```python
from build123d import *

# Parameters (mm, degrees)
SKETCH1_W           = 65
SKETCH1_H           = 30
BOSS_EXTRUDE1_DEPTH = 58
FILLET1_R           = 13
SKETCH15_W          = 83.696095513
SKETCH15_H          = 31.69844841
CUT_EXTRUDE7_DEPTH  = 50
SKETCH18_R          = 16
CUT_EXTRUDE10_DEPTH = 5.5
CUT_EXTRUDE12_REACH = 90.397
SKETCH3_R           = 1.6
SKETCH21_W          = 2
SKETCH21_H          = 2
CUT_EXTRUDE13_DEPTH = 8


with BuildPart() as part:
    # Sketch1 → Boss-Extrude1 (new body)
    with BuildSketch(Plane(origin=(0, 0, 0), x_dir=(1, 0, 0), z_dir=(0, 1, 0))):
        with Locations((7.5, 0)):
            Rectangle(SKETCH1_W, SKETCH1_H)
    extrude(amount=BOSS_EXTRUDE1_DEPTH)

    # Fillet1
    fillet1_edges = [part.edges().sort_by_distance(p)[0] for p in [
        (40, 29, 15),
        (-25, 29, 15),
        (-25, 29, -15),
        (40, 29, -15),
    ]]
    fillet(fillet1_edges, radius=FILLET1_R)

    # Sketch15 → Cut-Extrude7 (cut)
    with BuildSketch(Plane(origin=(0, -10, 0), x_dir=(-1, 0, 0), z_dir=(0, -1, 0))):
        with Locations((-0.057440767, 0.030479277)):
            Rectangle(SKETCH15_W, SKETCH15_H)
    extrude(amount=-CUT_EXTRUDE7_DEPTH, mode=Mode.SUBTRACT)

    # Sketch18 → Cut-Extrude10 (cut)
    with BuildSketch(Plane(origin=(0, 58, 0), x_dir=(1, 0, 0), z_dir=(0, 1, 0))):
        with Locations((6.828508286, 0)):
            Circle(SKETCH18_R)
    extrude(amount=-CUT_EXTRUDE10_DEPTH, mode=Mode.SUBTRACT)

    # Sketch3 → Cut-Extrude12 (cut, up to next)
    with BuildSketch(Plane.ZY.offset(25), mode=Mode.PRIVATE) as cut_extrude12_sk1:
        with Locations((0, 50.4)):
            Circle(SKETCH3_R)
    cut_extrude12_tool1 = extrude(cut_extrude12_sk1.sketch, amount=-CUT_EXTRUDE12_REACH, mode=Mode.PRIVATE) & part.part
    add(cut_extrude12_tool1.solids().sort_by_distance((-25, 50.4, 0))[0], mode=Mode.SUBTRACT)

    # Sketch21 → Cut-Extrude13 (cut)
    with BuildSketch(Plane(origin=(0, 52.5, 0), x_dir=(1, 0, 0), z_dir=(0, 1, 0))):
        with Locations((6.828508286, 0)):
            Rectangle(SKETCH21_W, SKETCH21_H)
    extrude(amount=-CUT_EXTRUDE13_DEPTH, mode=Mode.SUBTRACT)

    # Sketch24 → Revolve1 (revolve)
    with BuildSketch(Plane.XY, mode=Mode.PRIVATE) as revolve1_sk:
        Polygon((-25, 51), (-25, 52.4), (-35, 51), align=None)
    revolve(revolve1_sk.sketch.rotate(Axis((-25, 50.4, 0), (-1, 0, 0)), 90), axis=Axis((-25, 50.4, 0), (-1, 0, 0)))

    # Sketch25 → Revolve2 (revolve)
    with BuildSketch(Plane.XY, mode=Mode.PRIVATE) as revolve2_sk:
        Polygon((39.995235715, 52.4), (49.995235715, 51), (39.995235715, 51), align=None)
    revolve(revolve2_sk.sketch.rotate(Axis((-25, 50.4, 0), (1, 0, 0)), 90), axis=Axis((-25, 50.4, 0), (1, 0, 0)))


solid = part.part
```
Here's how the part is built. I have some questions about the finished solid (model axes, mm). A direction names the side the tool comes from. Round coordinates to 2 decimals unless told otherwise and drop trailing zeros. Order: outer loops, then holes, each group sorted by start corner. A loop starts at its lowest first (then second) coordinate and runs counter-clockwise, first axis right, second up. Notation, with made-up numbers: M 8.25,-8 L 67.25,-8 A29 cw 67.25,19 Z; hole C 18,22.25 d11. An arc over 180 degrees is marked long. One line per question, with ' | ' between items.
1) For pin 1 Ø1 at (y, z) = (46, 0) entering from -X; pin 2 Ø2 at (y, z) = (45.5, -1) entering from +X; pin 3 Ø1 at (y, z) = (49.5, 0) entering from -X; pin 4 Ø10 at (x, y) = (-23, 43) entering from -Z, each with a flat end and sliding along its axis, tell me the tip position at first contact or that it passes through.
Working result:
pin 1: x = -25 | pin 2: x = 40 | pin 3: x = -35 | pin 4: z = -13.53
2) For faces 5 (the face through (-15, 58, 0)), 6 (the face through (-25, 50, 1)), 7 (the face through (7.829, 47, 0)), which set-ups out of +Z, -Z, +X, -X, +Y, -Y let a thin tool reach every point of the face, with its end or its side?
Working result:
face 5: +Z, -Z, +X, -X, +Y | face 6: none | face 7: +Y
3) If we mould it in two halves opening along X, with no side actions, what happens to faces 1 (the face through (7, 52.5, -4)), 2 (the face through (36.091, 49.126, 11.293)), 3 (the face through (-21.293, 49.126, 11.091)), 4 (the face through (7, 49, 15))? For each: +X half, -X half, draft (parallel to the pull), parting line (faces both ways), or undercut.
Working result:
face 1: undercut | face 2: +X half | face 3: -X half | face 4: draft
4) I want a section at D-D, the plane z = 12. Write out the boundary of the cut face in (x, y), then the cut area to 3 significant figures.
Working result:
outline: M -20.31,40 L 35.31,40 L 35.31,58 L 17.41,58 L 17.41,52.5 L -3.75,52.5 L -3.75,58 L -20.31,58 Z | area: 885 mm²
5) I want a section at C-C, the plane y = 42.25. Write out the boundary of the cut face in (x, z).
Working result:
outline: M -25,-2 A13 ccw -12,-15 L 27,-15 A13 ccw 40,-2 L 40,2 A13 ccw 27,15 L -12,15 A13 ccw -25,2 Z
6) I want a section at B-B, the plane x = 17.5. Write out the boundary of the cut face in (y, z).
Working result:
outline: M 40,-15 L 58,-15 L 58,-11.92 L 52.5,-11.92 L 52.5,11.92 L 58,11.92 L 58,15 L 40,15 Z; hole C 50.4,0 d3.2
7) I want a section at A-A, the plane y = 55. Write out the boundary of the cut face in (x, z).
Working result:
outline: M -25,-2 A13 ccw -12,-15 L 1.26,-15 A16 cw 1.26,15 L -12,15 A13 ccw -25,2 Z; M 12.4,-15 L 27,-15 A13 ccw 40,-2 L 40,2 A13 ccw 27,15 L 12.4,15 A16 cw Z
8) I need wall thicknesses on line 1 along Y through (x, z) = (-10, 0); line 2 along Y through (x, z) = (-9, 0); line 3 along Y through (x, z) = (-4, 7.5). Which ranges of each line are inside material? Lowest first, please.
Working result:
line 1: 40 to 48.8, 52 to 58 | line 2: 40 to 48.8, 52 to 52.5 | line 3: 40 to 52.5
